Autodesk Fusion 360 part; units mm, degrees
sketch "LampBase" plane through (0, 0, 0) normal (0, 0, 1) x (1, 0, 0)
  line L0 (0, 0) -> (125, 0)
  line L1 (125, 0) -> (125, 32)
  line L2 (125, 32) -> (0, 32)
  line L3 (0, 32) -> (0, 0)
  dimension "d1" = 125
  dimension "d2" = 32
revolve "Revolve1" add sketch "LampBase" angle 360 about axis through (0, 32, 0) along (0, -1, 0)
fillet "Fillet1" radius 15 1 edges at (-116.5409, 32, -45.2019)
shell "Shell1" thickness 5 removed faces 1 at (-15.2225, 0, 33.3824)
sketch "Sketch2" plane through (0, 32, 0) normal (0, 1, 0) x (-1, 0, 0)
  circle A0 centre (0, 0) radius 110
  circle A1 centre (85, 0) radius 10
  dimension "d6" = 20
  dimension "d7" = 85
extrude "Extrude1" cut sketch "Sketch2" against normal blind 10 contours A1
The listing builds one solid part. Answer for the finished solid, in the listing's coordinates (mm). A direction names the side the tool comes from. Round coordinates to 2 decimals unless told otherwise and drop trailing zeros. Loops run counter-clockwise (first coordinate to the right, second up) from the corner with the lowest first, then second, coordinate; pieces in that order, holes last.
Q1. Given pin 1 Ø6 at (x, y) = (-80.5, 26.5) entering from -Z; pin 2 Ø5 at (x, z) = (-7.5, -9) entering from -Y; pin 3 Ø4 at (y, z) = (27, 65.5) entering from -X, each flat-ended and moving along its own axis, determine where each tip first touches the part or whether it passes through.
Q2. Section B-B, the plane x = 0 is taken. Determine the outline of the cut face in (y, z), then the cut area to 3 significant figures.
Q3. Find the intervals of material crossed by line 1 (Z direction, x = 0, y = 12); line 2 (Y direction, x = 107.5, z = -2); line 3 (X direction, y = 16.5, z = 101), in increasing order.
Q4. For a pull along X with two mould halves and no side action, classify faces 1 (the face through (-124.88, 8.62, -5.5)), 2 (the face through (-119.884, 8.619, -5.276)), 3 (the face through (-2, 32, 2)) as released by +X, released by -X, zero draft, split by the parting line, or undercut.
Q5. Section C-C, the plane y = 5 is taken. Determine the outline of the cut face in (x, z), then the cut area to 3 significant figures.
Q6. Which of the six approach directions +Z, -Z, +X, -X, +Y, -Y give full straight-line access (tool end or side, diameter ignored) to faces 4 (the face through (-2, 27, 2)), 5 (the face through (-75, 30, 0))?
Q7. Section A-A, the plane z = 0 is taken. Determine the outline of the cut face in (x, y).
Completed:
1. pin 1: stops at z = -94.88
1. pin 2: stops at y = 27
1. pin 3: stops at x = -104.18
2. outline: (0, -125) - (17, -125) arc R15 ccw to (32, -110) - (32, 110) arc R15 ccw to (17, 125) - (0, 125) - (0, 120) - (17, 120) arc R10 cw to (27, 110) - (27, -110) arc R10 cw to (17, -120) - (0, -120) - close
2. area: 1,470 mm2
3. line 1: z = -125 to -120, 120 to 125
3. line 2: y = 27 to 32
3. line 3: x = -73.65 to -64.8, 64.8 to 73.65
4. face 1: split by the parting line
4. face 2: undercut
4. face 3: zero draft
5. outline: circle Ø250 at (0, 0); hole circle Ø240 at (0, 0)
5. area: 3,850 mm2
6. face 4: -Y
6. face 5: +Y, -Y
7. outline: (-125, 0) - (-120, 0) - (-120, 17) arc R10 cw to (-110, 27) - (-95, 27) - (-95, 32) - (-110, 32) arc R15 ccw to (-125, 17) - close; (-75, 27) - (110, 27) arc R10 cw to (120, 17) - (120, 0) - (125, 0) - (125, 17) arc R15 ccw to (110, 32) - (-75, 32) - close
